Design review of the part built by this model. Coordinates are the model's own, in mm. A direction names the side the tool comes from. Coordinates: 2 decimals unless noted, no trailing zeros. Loops run counter-clockwise (first coordinate to the right, second up) from the corner with the lowest first, then second, coordinate; pieces in that order, holes last.
from build123d import *

# Parameters (mm, degrees)
SKETCH_1_R      = 1.6
SKETCH_1_R_2    = 3.1
EXTRUDE_1_DEPTH = 3
FILLET_1_R      = 1.6


with BuildPart() as part:
    # 草图1 → 凸台-拉伸1 (new body)
    with BuildSketch(Plane(origin=(0, 0, 0), x_dir=(1, 0, 0), z_dir=(0, 1, 0))):
        with BuildLine():
            Line((20.346167364, 17.486665594), (1.461595535, 18.943699177))
            ThreePointArc((1.461595535, 18.943699177), (-4.422619767, 18.478106894), (-9.88, 16.229158943))
            Line((-9.88, 16.229158943), (-28.12, 5.124997561))
            ThreePointArc((-28.12, 5.124997561), (-30.999566723, 0.072105046), (-28.242269316, -5.048533419))
            Line((-28.242269316, -5.048533419), (-25.544130748, -6.781332069))
            Line((-25.544130748, -6.781332069), (-28.786400064, -11.829865488))
            ThreePointArc((-28.786400064, -11.829865488), (-27.431701987, -18.047967539), (-21.213599936, -16.693269462))
            Line((-21.213599936, -16.693269462), (-17.97133062, -11.644736044))
            Line((-17.97133062, -11.644736044), (-0.301463654, -22.992678651))
            Line((-0.301463654, -22.992678651), (-3.543732971, -28.04121207))
            ThreePointArc((-3.543732971, -28.04121207), (-2.189034894, -34.259314121), (4.029067158, -32.904616044))
            Line((4.029067158, -32.904616044), (7.271336474, -27.856082626))
            Line((7.271336474, -27.856082626), (16.97889821, -8.527427253))
            ThreePointArc((16.97889821, -8.527427253), (17.476097582, -7.455602812), (17.905715537, -6.35494698))
            Line((17.905715537, -6.35494698), (24.240827364, 11.494880978))
            ThreePointArc((24.240827364, 11.494880978), (23.772996273, 15.452447578), (20.346167364, 17.486665594))
        make_face()
        Polygon((-12.211829252, -9.383402127), (-15.291662532, -2), (-4.828427125, -2), align=None, mode=Mode.SUBTRACT)
        Polygon((-15.270134549, 2), (-12.227051834, 9.398624709), (-4.828427125, 2), align=None, mode=Mode.SUBTRACT)
        Polygon((-9.383402127, 12.211829252), (-2, 15.291662532), (-2, 4.828427125), align=None, mode=Mode.SUBTRACT)
        Polygon((2, 15.270134549), (9.398624709, 12.227051834), (2, 4.828427125), align=None, mode=Mode.SUBTRACT)
        Polygon((12.211829252, 9.383402127), (15.291662532, 2), (4.828427125, 2), align=None, mode=Mode.SUBTRACT)
        Polygon((15.270134549, -2), (12.227051834, -9.398624709), (4.828427125, -2), align=None, mode=Mode.SUBTRACT)
        Polygon((9.383402127, -12.211829252), (2, -15.291662532), (2, -4.828427125), align=None, mode=Mode.SUBTRACT)
        Polygon((-2, -15.270134549), (-9.398624709, -12.227051834), (-2, -4.828427125), align=None, mode=Mode.SUBTRACT)
        with Locations(Location((20, 13, 0), (0, 0, 270))):
            Circle(SKETCH_1_R, mode=Mode.SUBTRACT)
        with BuildLine():
            Line((-25, 1.6), (-23, 1.6))
            ThreePointArc((-23, 1.6), (-21.4, 0), (-23, -1.6))
            Line((-23, -1.6), (-25, -1.6))
            ThreePointArc((-25, -1.6), (-26.6, 0), (-25, 1.6))
        make_face(mode=Mode.SUBTRACT)
        with Locations(Location((0.242667093, -30.472914057, 0), (0, 0, 270))):
            Circle(SKETCH_1_R, mode=Mode.SUBTRACT)
        with Locations(Location((-25, -14.261567475, 0), (0, 0, 270))):
            Circle(SKETCH_1_R, mode=Mode.SUBTRACT)
        with Locations(Location((0, 0, 0), (0, 0, 270))):
            Circle(SKETCH_1_R_2, mode=Mode.SUBTRACT)
    extrude(amount=EXTRUDE_1_DEPTH)

    # 圆角1
    fillet_1_edges = [part.edges().sort_by_distance(p)[0] for p in [
        (15.291662532, 1.5, -2),
        (12.211829252, 1.5, -9.383402127),
        (4.828427125, 1.5, -2),
        (9.398624709, 1.5, -12.227051834),
        (2, 1.5, -15.270134549),
        (2, 1.5, -4.828427125),
        (-2, 1.5, -15.291662532),
        (-9.383402127, 1.5, -12.211829252),
        (-2, 1.5, -4.828427125),
        (-12.227051834, 1.5, -9.398624709),
        (-15.270134549, 1.5, -2),
        (-4.828427125, 1.5, -2),
        (-15.291662532, 1.5, 2),
        (-12.211829252, 1.5, 9.383402127),
        (-9.398624709, 1.5, 12.227051834),
        (-2, 1.5, 15.270134549),
        (-2, 1.5, 4.828427125),
        (2, 1.5, 15.291662532),
        (9.383402127, 1.5, 12.211829252),
        (2, 1.5, 4.828427125),
        (12.227051834, 1.5, 9.398624709),
        (15.270134549, 1.5, 2),
        (4.828427125, 1.5, 2),
        (-0.301463654, 1.5, 22.992678651),
        (-17.97133062, 1.5, 11.644736044),
        (-25.544130748, 1.5, 6.781332069),
    ]]
    fillet(fillet_1_edges, radius=FILLET_1_R)


solid = part.part
Q1. Take a section at A-A, the plane z = 31. Write out the cut boundary in (x, y).
Q2. Clearance check with flat-ended pins moving along their axes: pin 1 Ø1.5 at (x, y) = (-11.5, 1) entering from -Z; pin 2 Ø1.5 at (y, z) = (1, 10.5) entering from +X; pin 3 Ø1.5 at (x, y) = (11, 1) entering from +Z. State where each tip first meets the part, or that it passes through.
Q3. Take a section at B-B, the plane z = 0. Write out the cut boundary in (x, y), then the cut area to 3 significant figures.
Q4. For line 1 (X direction, y = 0.25, z = 9); line 2 (X direction, y = 2.6, z = 7.5); line 3 (X direction, y = 2.05, z = -9), list the stretches that pass through material, from the lowest coordinate up.
Q5. The part is to be moulded in two halves that separate along Z. For faces 1 (the cylindrical face through (14.21, 1.521, -2.695)), 2 (the flat face through (12.057, 1.479, 18.327)), 3 (the cylindrical face through (-2.272, 1.479, 34.205)), 4 (the flat face through (-4, 0, 2)), say which applies: pulls with the +Z half, pulls with the -Z half, needs draft (parallel to the pull), parting line crosses it, or undercut.
Q6. Machinability: for faces 5 (the flat face through (-20.041, 1.479, 14.868)), 6 (the flat face through (-13.76, 1.48, -5.67)), which of the approach directions +Z, -Z, +X, -X, +Y, -Y give a long, thin tool a straight path to every point of the face, cutting with its end or side? Answer none if there is none.
Q7. Take a section at D-D, the plane y = 1.7. Give the number of separate pieces and of enclosed holes in the cut face, then the cut area to 3 significant figures.
Q8. Take a section at C-C, the plane x = -20.5. Write out the cut boundary in (y, z), then the cut area to 3 significant figures.
Entries:
1. outline: (-4.23, 0) - (-1.27, 0) - (-1.27, 3) - (-4.23, 3) - close; (1.75, 0) - (5.25, 0) - (5.25, 3) - (1.75, 3) - close
2. pin 1: stops at z = -15.7
2. pin 2: stops at x = 16.36
2. pin 3: stops at z = 21.93
3. outline: (-31, 0) - (-26.6, 0) - (-26.6, 3) - (-31, 3) - close; (-21.4, 0) - (-3.1, 0) - (-3.1, 3) - (-21.4, 3) - close; (3.1, 0) - (20.16, 0) - (20.16, 3) - (3.1, 3) - close
3. area: 119 mm2
4. line 1: x = -26.97 to -6.17, -2 to 2, 6.17 to 16.74
4. line 2: x = -26.17 to -12.95, -10.33 to -4.67, -2.53 to 2.53, 4.67 to 10.33, 12.96 to 17.46
4. line 3: x = -21.75 to -6.17, -2 to 2, 6.17 to 23.36
5. face 1: undercut
5. face 2: pulls with the +Z half
5. face 3: undercut
5. face 4: needs draft
6. face 5: +Z, +Y, -Y
6. face 6: +Y, -Y
7. separate pieces: 1
7. enclosed holes: 13
7. area: 1,420 mm2
8. outline: (0, -9.76) - (3, -9.76) - (3, 15.58) - (0, 15.58) - close
8. area: 76.0 mm2
